Model file for the job. Use its own axes, mm. Face numbers are marked on the shaded views. A direction names the side the tool comes from. Round coordinates to 2 decimals unless told otherwise and drop trailing zeros. Write each loop counter-clockwise with the first axis right and the second up, starting at its lowest first coordinate (ties: lowest second). Pieces come first, ordered by that corner, then holes. Notation, with made-up numbers: (-6.5, -3) - (6.5, -3) arc R32 ccw to (6.5, 30) - close; hole circle Ø8 at (88.25, -21). An arc over 180 degrees is marked (long way). One line per item, written item: value.
from build123d import *

# Parameters (mm, degrees)
BOSS_EXTRUDE1_DEPTH = 13.5
CUT_EXTRUDE1_DEPTH  = 13.5


with BuildPart() as part:
    # Sketch1 → Revolve1 (revolve)
    with BuildSketch(Plane.XY):
        with BuildLine():
            Line((0, 0), (0, -6.5))
            Line((0, -6.5), (85, -6.5))
            Line((85, -6.5), (125, -3))
            Line((125, -3), (149.222035298, -3))
            Line((149.222035298, -3), (149.222035298, -2))
            Line((149.222035298, -2), (150.222035298, -2))
            Line((150.222035298, -2), (150.222035298, -3))
            Line((150.222035298, -3), (156.707023179, -3))
            ThreePointArc((156.707023179, -3), (158.934336378, -2.137547522), (160, 0))
            Line((160, 0), (0, 0))
        make_face()
    revolve(axis=Axis((0, 0, 0), (1, 0, 0)))

    # Sketch2 → Boss-Extrude1 (add)
    with BuildSketch(Plane.ZY):
        with BuildLine():
            Line((-2.658777536, 5.931349089), (-2.658777536, -5.931349089))
            ThreePointArc((-2.658777536, -5.931349089), (0, -6.5), (2.658777536, -5.931349089))
            Line((2.658777536, -5.931349089), (2.658777536, 5.931349089))
            ThreePointArc((2.658777536, 5.931349089), (0, 6.5), (-2.658777536, 5.931349089))
        make_face()
    extrude(amount=BOSS_EXTRUDE1_DEPTH)

    # Sketch3 → Cut-Extrude1 (cut)
    with BuildSketch(Plane.XY.offset(2.658777536)):
        with BuildLine():
            Line((-7.271115967, 6.669291611), (-14.242543504, 7.619628139))
            Line((-14.242543504, 7.619628139), (-14.81279281, -7.656627724))
            Line((-14.81279281, -7.656627724), (-6.247435847, -8.529121085))
            Line((-6.247435847, -8.529121085), (-7.632896548, -6.659471856))
            ThreePointArc((-7.632896548, -6.659471856), (-13.535199526, 0.170025059), (-7.271115967, 6.669291611))
        make_face()
    extrude(amount=-CUT_EXTRUDE1_DEPTH, mode=Mode.SUBTRACT)


solid = part.part
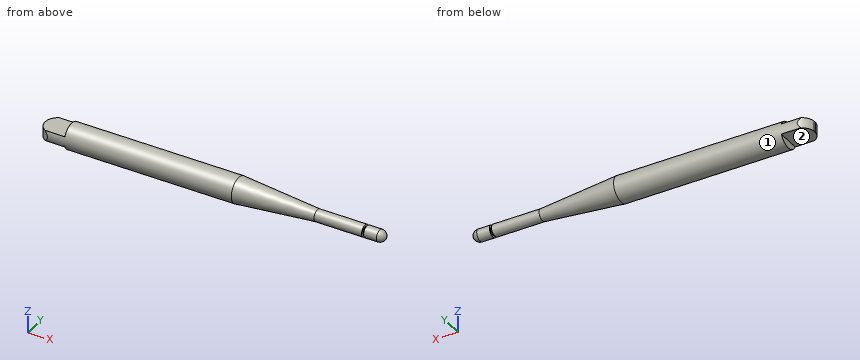
1. Wall check: probe 1 along Y at (x, z) = (38.5, 5.75); probe 2 along Y at (x, z) = (67, 0.5); probe 3 along Z at (x, y) = (-3, -0.5). Give the ranges that are in metal, low to high. Write a range as [from, to].
Report:
probe 1: [-3.03, 3.03]
probe 2: [-6.48, 6.48]
probe 3: [-2.66, 2.66]
2. Tool access for the marked faces 1 and 2: list every direction of +Z, -Z, +X, -X, +Y, -Y with a clear straight run to the whole face (end or side of a thin tool).
Report:
face 1: +X, -X
face 2: -Z, -X, +Y, -Y
3. Band-saw the part on B-B on x = 130. Write the cut outline in (y, z).
Report:
outline: circle Ø6 at (0, 0)
4. Band-saw the part on A-A on x = 58. Write the cut outline in (y, z), plus the area to 3 significant figures.
Report:
outline: circle Ø13 at (0, 0)
area: 133 mm²
5. Drop flat-ended pins along their axis: pin 1 (6 mm diameter, centred on x = 122, z = -3.5, fed in from +Y); pin 2 (6 mm diameter, centred on x = -9, y = 1.5, fed in from -Z); pin 3 (5 mm diameter, centred on y = 2.5, z = 2, fed in from +X); pin 4 (5 mm diameter, centred on y = -1, z = 0.5, fed in from -X). Give the stop position or say it passes through.
Report:
pin 1: y = 3.28
pin 2: z = -2.66
pin 3: x = 159.86
pin 4: x = -13.5
